from build123d import *

# Parameters (mm, degrees)
SKETCH1_W           = 25.4
SKETCH1_H           = 3.048
BOSS_EXTRUDE1_DEPTH = 10.16
SKETCH2_W           = 30.48
SKETCH2_H           = 6.35
BOSS_EXTRUDE2_DEPTH = 3.175
FILLET1_R           = 1.27


with BuildPart() as part:
    # Sketch1 → Boss-Extrude1 (new body)
    with BuildSketch(Plane(origin=(0, 0, 0), x_dir=(1, 0, 0), z_dir=(0, 1, 0))):
        Rectangle(SKETCH1_W, SKETCH1_H)
    extrude(amount=BOSS_EXTRUDE1_DEPTH)

    # Sketch2 → Boss-Extrude2 (add)
    with BuildSketch(Plane.XZ):
        Rectangle(SKETCH2_W, SKETCH2_H)
    extrude(amount=BOSS_EXTRUDE2_DEPTH)

    # Fillet1
    fillet1_edges = [part.edges().sort_by_distance(p)[0] for p in [
        (-12.7, 10.16, 0),
        (15.24, 0, 0),
        (15.24, -1.5875, -3.175),
        (0, 0, 3.175),
        (15.24, -1.5875, 3.175),
        (-15.24, 0, 0),
        (-15.24, -1.5875, 3.175),
        (0, 0, -3.175),
        (-15.24, -1.5875, -3.175),
        (15.24, -3.175, 0),
        (0, -3.175, 3.175),
        (-15.24, -3.175, 0),
        (0, 10.16, 1.524),
        (0, -3.175, -3.175),
        (12.7, 5.08, 1.524),
        (-12.7, 5.08, 1.524),
        (-12.7, 5.08, -1.524),
        (12.7, 5.08, -1.524),
        (0, 10.16, -1.524),
    ]]
    fillet(fillet1_edges, radius=FILLET1_R)


solid = part.part
Can you work these out from the model? Positions are in its coordinate system, mm. A direction names the side the tool comes from. Give positions to 0.01 mm unless a question says otherwise; leave off trailing zeros. Loops run counter-clockwise (first coordinate to the right, second up) from the corner with the lowest first, then second, coordinate; pieces in that order, holes last. Notation, with made-up numbers: (-10.75, 32.25) -> (19.25, 32.25) arc R26 ccw to (19.25, 58.25) -> close; hole circle Ø11 at (35, -21.5). An arc over 180 degrees is marked (long way). Use one line per item in the form item = value.
1) I need wall thicknesses on line 1 along X through (y, z) = (4.5, 0.25); line 2 along Y through (x, z) = (13.5, -1.25) (3 decimals); line 3 along Z through (x, y) = (10, 6). Which ranges of each line are inside material? Lowest first, please.
Answers:
line_1 = -12.7 to 12.7
line_2 = -3.175 to 0
line_3 = -1.52 to 1.52
2) If we section it at A-A (x = -9): Please give me the cut outline in (y, z) (3 decimals).
Answers:
outline = (-3.175, -1.905) arc R1.27 ccw to (-1.905, -3.175) -> (-1.27, -3.175) arc R1.27 ccw to (0, -1.905) -> (0, -1.524) -> (8.89, -1.524) arc R1.27 ccw to (10.16, -0.254) -> (10.16, 0.254) arc R1.27 ccw to (8.89, 1.524) -> (0, 1.524) -> (0, 1.905) arc R1.27 ccw to (-1.27, 3.175) -> (-1.905, 3.175) arc R1.27 ccw to (-3.175, 1.905) -> close
3) Will these pins go through, and if not, where does the flat tip stop? pin 1 (3 mm diameter, centred on y = 4, z = -1.5, fed in from -X); pin 2 (1 mm diameter, centred on y = 6, z = -1, fed in from +X); pin 3 (1.5 mm diameter, centred on x = -7.5, y = 4, fed in from +Z).
Answers:
pin_1 = -12.7
pin_2 = 12.68
pin_3 = 1.52
4) For faces 1 (the face through (0, 4, 1.524)), 2 (the face through (-12.34, 4.51, 1.14)), 3 (the face through (12.32, 5.15, -1.16)), 4 (the face through (-12.34, 4.51, -1.14)), 5 (the face through (-0.1, 0, 1.7)), which set-ups out of +Z, -Z, +X, -X, +Y, -Y let a thin tool reach every point of the face, with its end or its side?
Answers:
face_1 = +Z, +X, -X, +Y
face_2 = +Z, -X, +Y
face_3 = -Z, +X, +Y
face_4 = -Z, -X, +Y
face_5 = +Y
5) If we section it at B-B (y = 5.75): Please give me the cut outline in (x, z), plus the area to 3 significant figures.
Answers:
outline = (-12.7, -0.25) arc R1.27 ccw to (-11.43, -1.52) -> (11.43, -1.52) arc R1.27 ccw to (12.7, -0.25) -> (12.7, 0.25) arc R1.27 ccw to (11.43, 1.52) -> (-11.43, 1.52) arc R1.27 ccw to (-12.7, 0.25) -> close
area = 76.0 mm²
6) If we section it at C-C (z = 1.25): Please give me the cut outline in (x, y) (3 decimals), plus the area to 3 significant figures.
Answers:
outline = (-15.24, -1.905) arc R1.27 ccw to (-13.97, -3.175) -> (13.97, -3.175) arc R1.27 ccw to (15.24, -1.905) -> (15.24, -1.27) arc R1.27 ccw to (13.97, 0) -> (12.218, 0) -> (12.218, 9.678) -> (-11.43, 9.678) arc R0.788 ccw to (-12.218, 8.89) -> (-12.218, 0) -> (-13.97, 0) arc R1.27 ccw to (-15.24, -1.27) -> close
area = 332 mm²
7) If we section it at D-D (y = 9.5): Please give me the cut outline in (x, z).
Answers:
outline = (-12.54, -0.25) arc R1.11 ccw to (-11.43, -1.37) -> (12.04, -1.37) arc R1.27 ccw to (12.7, -0.25) -> (12.7, 0.25) arc R1.27 ccw to (12.04, 1.37) -> (-11.43, 1.37) arc R1.11 ccw to (-12.54, 0.25) -> close
